```python
from build123d import *

# Parameters (mm, degrees)
BOSS_EXTRUDE1_DEPTH = 10
FILLET1_R           = 2
SKETCH2_W           = 21
SKETCH2_H           = 2.5
BOSS_EXTRUDE2_DEPTH = 20
SKETCH3_R           = 2.25
CUT_EXTRUDE1_DEPTH  = 108.274472732


with BuildPart() as part:
    # Sketch1 → Boss-Extrude1 (new body)
    with BuildSketch(Plane(origin=(0, 0, 0), x_dir=(0, 0, -1), z_dir=(1, 0, 0))):
        with BuildLine():
            Line((-45, -42.5), (40, -42.5))
            ThreePointArc((40, -42.5), (43.535533906, -41.035533906), (45, -37.5))
            Line((45, -37.5), (45, 37.5))
            ThreePointArc((45, 37.5), (43.535533906, 41.035533906), (40, 42.5))
            Line((40, 42.5), (-45, 42.5))
            ThreePointArc((-45, 42.5), (-87.5, 0), (-45, -42.5))
        make_face()
    extrude(amount=BOSS_EXTRUDE1_DEPTH)

    # Fillet1
    fillet1_edges = [part.edges().sort_by_distance(p)[0] for p in [
        (0, 42.5, 2.5),
        (0, 41.035533906, -43.535533906),
        (0, 0, -45),
        (0, -41.035533906, -43.535533906),
        (0, -42.5, 2.5),
        (0, 0, 87.5),
    ]]
    fillet(fillet1_edges, radius=FILLET1_R)

    # Sketch2 → Boss-Extrude2 (add)
    with BuildSketch(Plane.ZY):
        with Locations((12.5, 15)):
            Rectangle(SKETCH2_W, SKETCH2_H)
    boss_extrude2 = extrude(amount=BOSS_EXTRUDE2_DEPTH)

    # Mirror1: Boss-Extrude2 across plane
    add(boss_extrude2.mirror(Plane.ZX))

    # Sketch3 → Cut-Extrude1 (cut, through all)
    with BuildSketch(Plane(origin=(0, 16.25, 0), x_dir=(1, 0, 0), z_dir=(0, 1, 0))):
        with Locations(Location((-13, -12.5, 0), (0, 0, 270))):
            Circle(SKETCH3_R)
    extrude(amount=-CUT_EXTRUDE1_DEPTH, mode=Mode.SUBTRACT)


solid = part.part
```
For this review, take the finished solid that the model builds, in its own axes (mm). A direction names the side the tool comes from. Coordinates: 2 decimals unless noted, no trailing zeros. Order: outer loops, then holes, each group sorted by start corner. A loop starts at its lowest first (then second) coordinate and runs counter-clockwise, first axis right, second up. Notation, with made-up numbers: (-17, 68) -> (2, 68) arc R19 cw to (2, 83) -> close; hole circle Ø3 at (81.5, 80.25). An arc over 180 degrees is marked (long way). Use CSV: the item, a comma, the result in double quotes. Start each with the question number.
Item 1: We need section A-A, the plane x = -9. Give the boundary of the cut face in (y, z).
Item 2: Insertion check: pin 1 (2 mm diameter, centred on x = -13.5, y = -15.5, fed in from -Z); pin 2 (6 mm diameter, centred on x = -12.5, z = 10, fed in from -Y); pin 3 (2 mm diameter, centred on x = 0.5, z = -26, fed in from -Y). Each pin has a flat end and moves straight along its axis. Give the tip position at first contact, or say it passes through.
Item 3: We need section D-D, the plane x = 7. Give the boundary of the cut face in (y, z).
Item 4: We need section C-C, the plane y = 0. Give the boundary of the cut face in (x, z).
Item 5: Wall thickness on probe 1 along X at (y, z) = (-14.95, 12.5); probe 2 along Y at (x, z) = (-0.75, 18); probe 3 along X at (y, z) = (-11, 5.5): over which ranges is each line inside the solid? List them lowest first.
Item 6: We need section B-B, the plane z = 12.5. Give the boundary of the cut face in (x, y).
Item 7: For faces 1 (the face through (-10, -16.25, 12)), 2 (the face through (-10, -13.75, 12)), 3 (the face through (-10, 15, 2)), list the 3-axis set-ups (+Z, -Z, +X, -X, +Y, -Y) from which the entire face can be reached by the end or side of a thin tool; tool diameter is ignored.
Item 8: Draft analysis for pull direction X (two halves, no side actions). For faces 4 (the face through (10, 1, 22)), 5 (the face through (5.94, 41, -43.57)), 6 (the face through (-11.48, -14.98, 10.84)), state which applies: pulls with the +X half, pulls with the -X half, needs draft (parallel to the pull), parting line crosses it, or undercut.
Derived:
1,outline,"(-16.25, 2) -> (-13.75, 2) -> (-13.75, 23) -> (-16.25, 23) -> close; (13.75, 2) -> (16.25, 2) -> (16.25, 23) -> (13.75, 23) -> close"
2,pin 1,"stops at z = 2"
2,pin 2,"stops at y = -16.25"
2,pin 3,"stops at y = -42.44"
3,outline,"(-42.5, -40) arc R5 ccw to (-37.5, -45) -> (37.5, -45) arc R5 ccw to (42.5, -40) -> (42.5, 45) arc R42.5 ccw to (-42.5, 45) -> close"
4,outline,"(0, -43) arc R2 ccw to (2, -45) -> (10, -45) -> (10, 87.5) -> (2, 87.5) arc R2 ccw to (0, 85.5) -> close"
5,probe 1,"x = -20 to -15.25, -10.75 to 10"
5,probe 2,"y = -16.25 to -13.75, 13.75 to 16.25"
5,probe 3,"x = 0 to 10"
6,outline,"(-20, -16.25) -> (-15.25, -16.25) -> (-15.25, -13.75) -> (-20, -13.75) -> close; (-20, 13.75) -> (-15.25, 13.75) -> (-15.25, 16.25) -> (-20, 16.25) -> close; (-10.75, -16.25) -> (0, -16.25) -> (0, -40.5) arc R2 ccw to (2, -42.5) -> (10, -42.5) -> (10, 42.5) -> (2, 42.5) arc R2 ccw to (0, 40.5) -> (0, 16.25) -> (-10.75, 16.25) -> (-10.75, 13.75) -> (0, 13.75) -> (0, -13.75) -> (-10.75, -13.75) -> close"
7,face 1,"+Z, -Z, -X, -Y"
7,face 2,"+Z, -Z, -X"
7,face 3,"-Z, -X, +Y, -Y"
8,face 4,"pulls with the +X half"
8,face 5,"needs draft"
8,face 6,"undercut"
